The figure shows three views and two pictorial views of one solid part (mm, origin at its lowest corner). Answer the questions. A direction names the side the tool comes from. Round coordinates to 2 decimals unless told otherwise and drop trailing zeros. Loops run counter-clockwise (first coordinate to the right, second up) from the corner with the lowest first, then second, coordinate; pieces in that order, holes last. Notation, with made-up numbers: (6.5, 30) -> (24.5, 30) arc R25 ccw to (24.5, 61) -> close; hole circle Ø2 at (-9, 72). An arc over 180 degrees is marked (long way). Put each result on its own line as item: value.
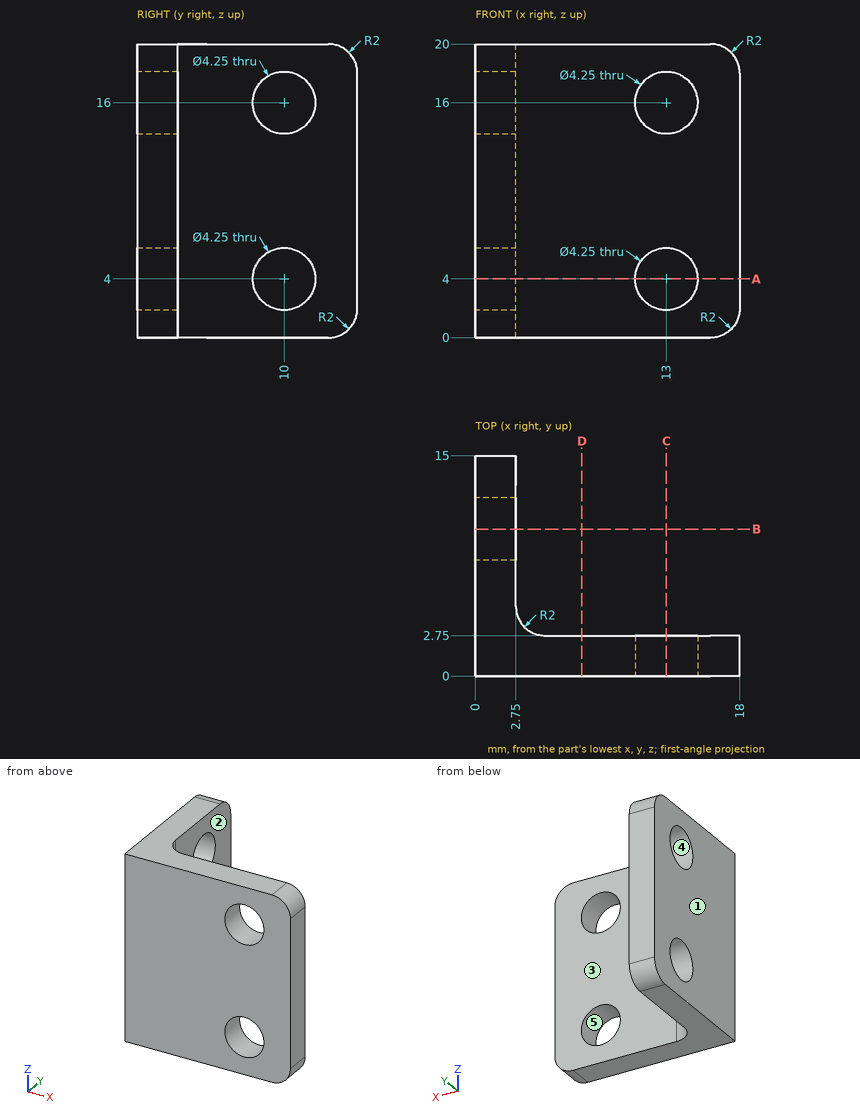
Item 1: The part is cut by section B-B (y = 10). Determine the outline of the cut face in (x, z) (3 decimals), then the cut area to 3 significant figures.
Derived:
outline: (0, 0) -> (2.75, 0) -> (2.75, 1.875) -> (0, 1.875) -> close; (0, 6.125) -> (2.75, 6.125) -> (2.75, 13.875) -> (0, 13.875) -> close; (0, 18.125) -> (2.75, 18.125) -> (2.75, 20) -> (0, 20) -> close
area: 31.6 mm^2
Item 2: For a pull along Y with two mould halves and no side action, classify the marked faces 3, 4 and 5 as pulls with the +Y half, pulls with the -Y half, needs draft (parallel to the pull), parting line crosses it, or undercut.
Derived:
face 3: pulls with the +Y half
face 4: undercut
face 5: needs draft
Item 3: The part is cut by section A-A (z = 4). Determine the outline of the cut face in (x, y) (3 decimals).
Derived:
outline: (0, 0) -> (10.875, 0) -> (10.875, 2.75) -> (4.75, 2.75) arc R2 cw to (2.75, 4.75) -> (2.75, 7.875) -> (0, 7.875) -> close; (0, 12.125) -> (2.75, 12.125) -> (2.75, 15) -> (0, 15) -> close; (15.125, 0) -> (18, 0) -> (18, 2.75) -> (15.125, 2.75) -> close
Item 4: The part is cut by section D-D (x = 7.25). Determine the outline of the cut face in (y, z).
Derived:
outline: (0, 0) -> (2.75, 0) -> (2.75, 20) -> (0, 20) -> close
Item 5: Flat-ended cylindrical pins translate along their axes: pin 1 Ø8 at (x, z) = (16, 7) entering from +Y; pin 2 Ø3 at (y, z) = (12, 10.5) entering from +X. Find the tip coordinate at first contact, or state that the pin passes through.
Derived:
pin 1: stops at y = 2.75
pin 2: stops at x = 2.75
Item 6: Which of the six approach directions +Z, -Z, +X, -X, +Y, -Y give full straight-line access (tool end or side, diameter ignored) to the marked faces 1 and 2?
Derived:
face 1: +Z, -Z, -X, +Y, -Y
face 2: +Z, -Z, +X, +Y
Item 7: Find the intervals of material crossed by line 1 along Y through (x, z) = (1.45, 16) (3 decimals); line 2 along X through (y, z) = (1.7, 4) (3 decimals); line 3 along X through (y, z) = (10, 19.25), in increasing order.
Derived:
line 1: y = 0 to 7.875, 12.125 to 15
line 2: x = 0 to 10.875, 15.125 to 18
line 3: x = 0 to 2.75
